Answer from the drawing. Dimensions are ordinates in mm from the lowest x, y and z of the part. Coordinates: 2 decimals unless noted, no trailing zeros. Order: outer loops, then holes, each group sorted by start corner. A loop starts at its lowest first (then second) coordinate and runs counter-clockwise, first axis right, second up. Notation, with made-up numbers: (-3.75, 58.5) -> (37.25, 58.5) arc R15 cw to (37.25, 87.5) -> close; hole circle Ø7 at (20, -9.75). An arc over 180 degrees is marked (long way). Answer in a Markdown table with one row per item.
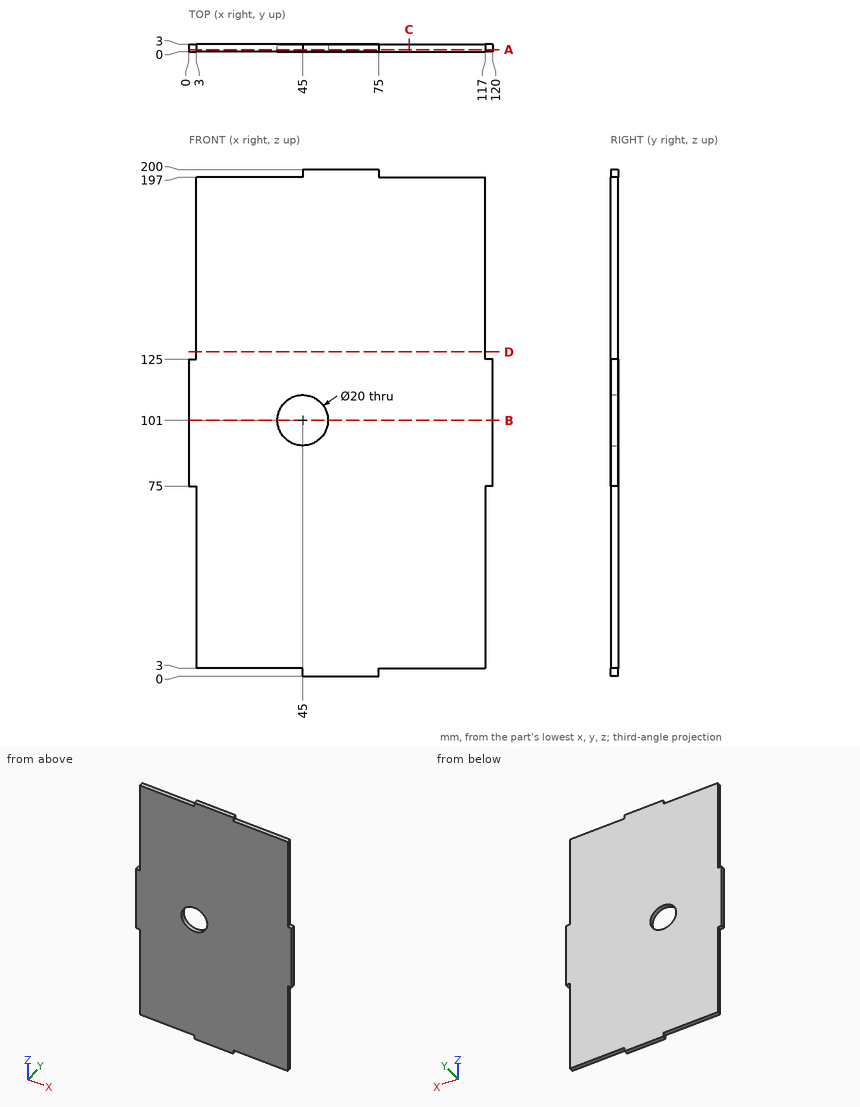
(1) A cutting plane is placed at C-C, the plane x = 87. Determine the outline of the cut face in (y, z), then the cut area to 3 significant figures.
Check values:
| item | result |
|---|---|
| outline | (0, 3) -> (3, 3) -> (3, 197) -> (0, 197) -> close |
| area | 582 mm² |
(2) Flat-ended cylindrical pins translate along their axes: pin 1 (1.5 mm diameter, centred on x = 1.5, y = 1, fed in from -Z); pin 2 (1.5 mm diameter, centred on x = 97.5, y = 2, fed in from -Z); pin 3 (1.5 mm diameter, centred on y = 2, z = 172, fed in from -X); pin 4 (10 mm diameter, centred on x = 73, z = 159, fed in from -Y). Find the tip coordinate at first contact, or state that the pin passes through.
Check values:
| item | result |
|---|---|
| pin 1 | z = 75 |
| pin 2 | z = 3 |
| pin 3 | x = 3 |
| pin 4 | y = 0 |
(3) A cutting plane is placed at B-B, the plane z = 101. Determine the outline of the cut face in (x, y).
Check values:
| item | result |
|---|---|
| outline | (0, 0) -> (35, 0) -> (35, 3) -> (0, 3) -> close; (55, 0) -> (120, 0) -> (120, 3) -> (55, 3) -> close |
(4) Find the intervals of material crossed by line 1 along X through (y, z) = (1.05, 101); line 2 along Z through (x, y) = (45.5, 1.35); line 3 along X through (y, z) = (0.2, 29), in increasing order. Write a range as from..to.
Check values:
| item | result |
|---|---|
| line 1 | 0..35, 55..120 |
| line 2 | 0..91.01, 110.99..200 |
| line 3 | 3..117 |
(5) A cutting plane is placed at A-A, the plane y = 0.75. Determine the outline of the cut face in (x, z).
Check values:
| item | result |
|---|---|
| outline | (0, 75) -> (3, 75) -> (3, 3) -> (45, 3) -> (45, 0) -> (75, 0) -> (75, 3) -> (117, 3) -> (117, 75) -> (120, 75) -> (120, 125) -> (117, 125) -> (117, 197) -> (75, 197) -> (75, 200) -> (45, 200) -> (45, 197) -> (3, 197) -> (3, 125) -> (0, 125) -> close; hole circle Ø20 at (45, 101) |
(6) A cutting plane is placed at D-D, the plane z = 128. Determine the outline of the cut face in (x, y), then the cut area to 3 significant figures.
Check values:
| item | result |
|---|---|
| outline | (3, 0) -> (117, 0) -> (117, 3) -> (3, 3) -> close |
| area | 342 mm² |
